from build123d import *

# Parameters (mm, degrees)
CROQUIS1_R                = 5
SALIENTE_EXTRUIR1_DEPTH   = 15
TALADRO_ROSCADO_M81_D     = 6.8
TALADRO_ROSCADO_M81_DEPTH = 20
TALADRO_ROSCADO_M81_TIP   = 2.042926105


with BuildPart() as part:
    # Croquis1 → Saliente-Extruir1 (new body)
    with BuildSketch(Plane.XY):
        Polygon((-64.5, 42), (-56.5, 50), (64.5, 50), (64.5, -50), (-56.5, -50), (-64.5, -42), align=None)
        with Locations((-29.5, 30)):
            Circle(CROQUIS1_R, mode=Mode.SUBTRACT)
        with BuildLine():
            ThreePointArc((-18.148924408, -31.968968709), (-5.213281237, -28.130502249), (6.608289397, -21.625492122))
            ThreePointArc((6.608289397, -21.625492122), (7.839813422, -14.662493589), (0.876814889, -13.430969563))
            ThreePointArc((0.876814889, -13.430969563), (-9.068315962, -18.9034384), (-19.950682438, -22.13262447))
            ThreePointArc((-19.950682438, -22.13262447), (-23.967975543, -27.951675605), (-18.148924408, -31.968968709))
        make_face(mode=Mode.SUBTRACT)
    extrude(amount=SALIENTE_EXTRUIR1_DEPTH)

    # Taladro roscado M81
    with Locations(Plane(origin=(64.5, 0, 0), x_dir=(0, 0, -1), z_dir=(1, 0, 0))):
        with Locations((-7.5, 40), (-7.5, 0), (-7.5, -40)):
            Hole(TALADRO_ROSCADO_M81_D / 2, depth=TALADRO_ROSCADO_M81_DEPTH)
            with Locations((0, 0, -(TALADRO_ROSCADO_M81_DEPTH + TALADRO_ROSCADO_M81_TIP / 2))):  # 118° drill point
                Cone(0, TALADRO_ROSCADO_M81_D / 2, TALADRO_ROSCADO_M81_TIP, mode=Mode.SUBTRACT)


solid = part.part
Design review of the part built by this model. Coordinates are the model's own, in mm. A direction names the side the tool comes from. Coordinates: 2 decimals unless noted, no trailing zeros. Loops run counter-clockwise (first coordinate to the right, second up) from the corner with the lowest first, then second, coordinate; pieces in that order, holes last. Notation, with made-up numbers: M 22.25,-36.5 L 45.25,-36.5 A26 cw 45.25,-21.5 Z; hole C 66.25,79 d11. An arc over 180 degrees is marked long. Use one line per item in the form item = value.
(1) Consider section A-A (x = -29.5). Write out the cut boundary in (y, z), and give its area (3 significant figures).
Return value:
outline = M -50,0 L 25,0 L 25,15 L -50,15 Z; M 35,0 L 50,0 L 50,15 L 35,15 Z
area = 1,350 mm2
(2) Consider section B-B (y = 30). Write out the cut boundary in (x, z), and give its area (4 significant figures).
Return value:
outline = M -64.5,0 L -34.5,0 L -34.5,15 L -64.5,15 Z; M -24.5,0 L 64.5,0 L 64.5,15 L -24.5,15 Z
area = 1,785 mm2
(3) For faces 1 (the face through (54.36, -1.3, 10.64)), 2 (the face through (-5.388, -28.203, 7.395)), 3 (the face through (1, 1, 15)), list the 3-axis set-ups (+Z, -Z, +X, -X, +Y, -Y) from which the entire face can be reached by the end or side of a thin tool; tool diameter is ignored.
Return value:
face_1 = +X
face_2 = +Z, -Z
face_3 = +Z, +X, -X, +Y, -Y
(4) Clearance check with a flat-ended pin moving along its axis: P1, Ø5.5, axis at y = 40, z = 7.5, coming from the +X side. State where the tip first meets the part, or that it passes through.
Return value:
P1 = 44.11
(5) For line 1 along Y through (x, z) = (51, 7.5); line 2 along Z through (x, y) = (49, 40); line 3 along X through (y, z) = (-13.5, 2.75), list the stretches that pass through material, from the lowest coordinate up. Write a range as from..to.
Return value:
line_1 = -50..-43.4, -36.6..-3.4, 3.4..36.6, 43.4..50
line_2 = 0..4.1, 10.9..15
line_3 = -64.5..0.78, 6.7..64.5
(6) Draft analysis for pull direction X (two halves, no side actions). For faces 4 (the face through (-8.92, -18.84, 7.4)), 5 (the face through (42.812, -0.226, 6.955)), 6 (the face through (1, 1, 0)), 7 (the face through (-60.6, 45.9, 7.4)), state which applies: pulls with the +X half, pulls with the -X half, needs draft (parallel to the pull), parting line crosses it, or undercut.
Return value:
face_4 = undercut
face_5 = pulls with the +X half
face_6 = needs draft
face_7 = pulls with the -X half
